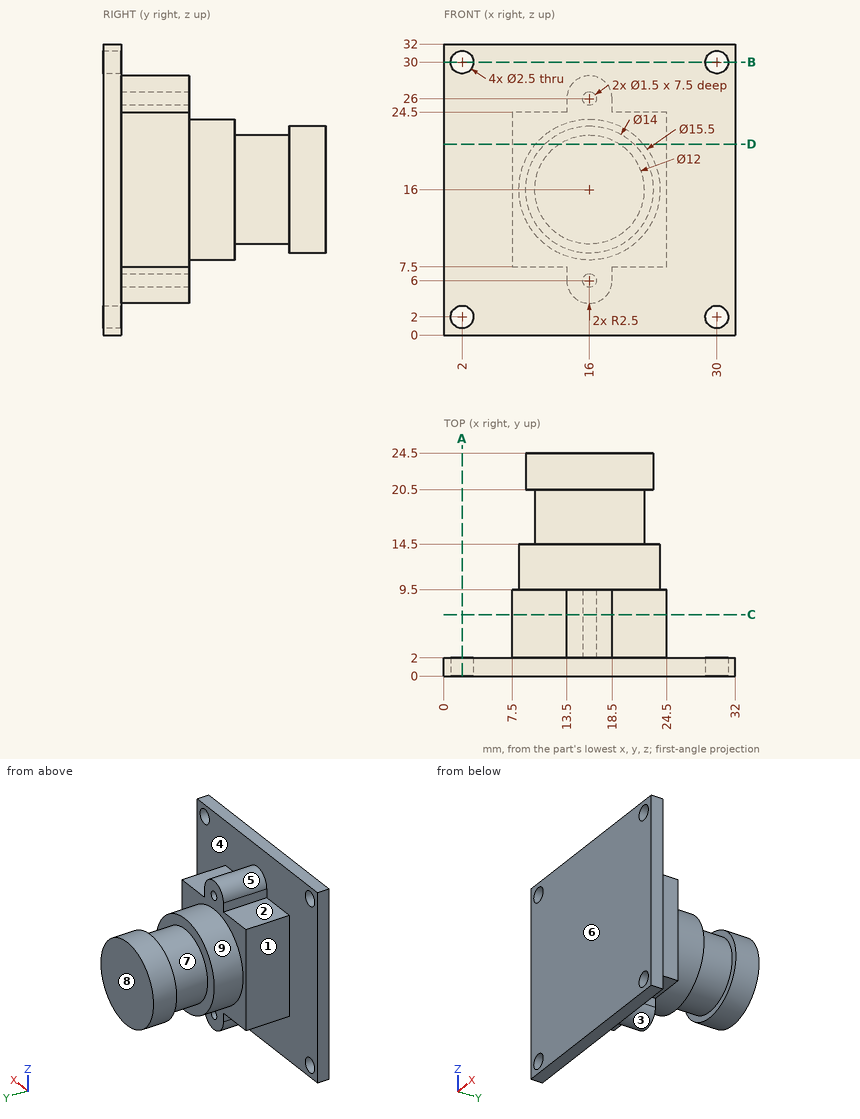
Source: three-view drawing plus pictorial views. Frame: mm from the lowest corner of the part. A direction names the side the tool comes from. Give positions to 0.01 mm unless a question says otherwise; leave off trailing zeros. Order: outer loops, then holes, each group sorted by start corner. A loop starts at its lowest first (then second) coordinate and runs counter-clockwise, first axis right, second up. Notation, with made-up numbers: M 33,-27.5 L 82,-27.5 A27 ccw 82,2.5 Z; hole C 61,21.25 d6. An arc over 180 degrees is marked long. Return JSON: item names as keys, results as strings.
1) Access query for the marked faces 1, 2, 3, 4 and 5. Directions: +Z, -Z, +X, -X, +Y, -Y. A direction counts if a zero-diameter tool reaches every point of the face in a straight line with its end or side. Return the directions, or none.
Taken from the geometry:
{"face 1": "+Z, -Z, -X, +Y", "face 2": "+Z, -X, +Y", "face 3": "-Z, +Y", "face 4": "+Y", "face 5": "+Z, +Y"}
2) Section query D-D on z = 21. Output: boundary loops of the cut face in (x, y), and give its area (3 significant figures).
Taken from the geometry:
{"outline": "M 0,0 L 32,0 L 32,2 L 24.5,2 L 24.5,9.5 L 21.92,9.5 L 21.92,14.5 L 19.32,14.5 L 19.32,20.5 L 20.9,20.5 L 20.9,24.5 L 11.1,24.5 L 11.1,20.5 L 12.68,20.5 L 12.68,14.5 L 10.08,14.5 L 10.08,9.5 L 7.5,9.5 L 7.5,2 L 0,2 Z", "area": "330 mm2"}
3) Section query A-A on x = 2. Output: boundary loops of the cut face in (y, z), and give its area (3 significant figures).
Taken from the geometry:
{"outline": "M 0,0 L 2,0 L 2,0.75 L 0,0.75 Z; M 0,3.25 L 2,3.25 L 2,28.75 L 0,28.75 Z; M 0,31.25 L 2,31.25 L 2,32 L 0,32 Z", "area": "54.0 mm2"}
4) Contact query for flat-ended pins moving along their axis: pin 1 (4 mm diameter, centred on x = 27, z = 22.5, fed in from -Y); pin 2 (6 mm diameter, centred on y = 6.5, z = 20.5, fed in from -X); pin 3 (1.6 mm diameter, centred on y = 7, z = 25.5, fed in from +X); pin 4 (6 mm diameter, centred on x = 6.5, z = 7.5, fed in from +Y). Output: stop coordinate, or through.
Taken from the geometry:
{"pin 1": "stops at y = 0", "pin 2": "stops at x = 7.5", "pin 3": "stops at x = 18.5", "pin 4": "stops at y = 9.5"}
5) Section query C-C on y = 6.75. Output: boundary loops of the cut face in (x, z).
Taken from the geometry:
{"outline": "M 7.5,7.5 L 13.5,7.5 L 13.5,6 A2.5 ccw 18.5,6 L 18.5,7.5 L 24.5,7.5 L 24.5,24.5 L 18.5,24.5 L 18.5,26 A2.5 ccw 13.5,26 L 13.5,24.5 L 7.5,24.5 Z; hole C 16,6 d1.5; hole C 16,26 d1.5"}
6) Mould query, pull axis Y, two halves, no side actions, for the marked faces 6, 7, 8 and 9. Classes: released by +Y, released by -Y, zero draft, split by the parting line, or undercut.
Taken from the geometry:
{"face 6": "released by -Y", "face 7": "undercut", "face 8": "released by +Y", "face 9": "zero draft"}
7) Line query: L1, parallel to X at y = 1.35, z = 30; L2, parallel to X at y = 7.5, z = 26; L3, parallel to Z at x = 16.5, y = 9.25. Output: solid intervals per line, ascending. Write a range as [from, to].
Taken from the geometry:
{"L1": "x = [0, 0.75], [3.25, 28.75], [31.25, 32]", "L2": "x = [13.5, 15.25], [16.75, 18.5]", "L3": "z = [3.55, 5.44], [6.56, 25.44], [26.56, 28.45]"}
8) Section query B-B on z = 30. Output: boundary loops of the cut face in (x, y), and give its area (3 significant figures).
Taken from the geometry:
{"outline": "M 0,0 L 0.75,0 L 0.75,2 L 0,2 Z; M 3.25,0 L 28.75,0 L 28.75,2 L 3.25,2 Z; M 31.25,0 L 32,0 L 32,2 L 31.25,2 Z", "area": "54.0 mm2"}
